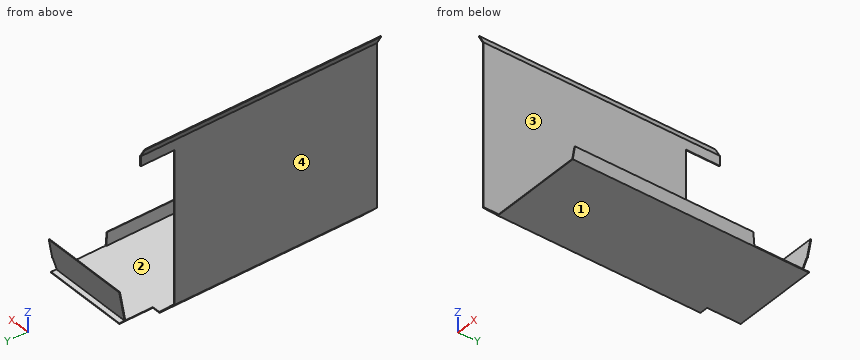
from build123d import *

# Parameters (mm, degrees)
F1_DEPTH  = 1076
F2_W      = 123
F2_H      = 775
F3_DEPTH  = 153
F5_DEPTH  = 402
F7_DEPTH  = 25
F9_DEPTH  = 50
F11_DEPTH = 260


with BuildPart() as f1:
    # F0 (on Front) → F1 (new body)
    with BuildSketch(Plane.XZ):
        Polygon((0, 819), (0, 85), (85, 0), (512, 0), (525, 50), (521.9029679783, 50.8052283256), (509.5256086136, 3.2), (86.3254833996, 3.2), (3.2, 86.3254833996), (3.2, 819.8498061986), (-21.2216219452, 862.5876446027), (-24, 861), align=None)
    extrude(amount=F1_DEPTH)

    # F2 (on face) → F3 (cut)
    with BuildSketch(Plane(origin=(0, 0, 0), x_dir=(-1, 0, 0), z_dir=(0, 1, 0))):
        with Locations((-61.5, 387.5)):
            Rectangle(F2_W, F2_H)
    extrude(amount=-F3_DEPTH, mode=Mode.SUBTRACT)

    # F4 (on face) → F5 (join)
    with BuildSketch(Plane(origin=(123, 0, 0), x_dir=(0, -1, 0), z_dir=(-1, 0, 0))):
        Polygon((0, 140), (25, 0), (28.1501682416, 0.5625300431), (3.1501682416, 140.5625300431), align=None)
    extrude(amount=-F5_DEPTH)

    # F6 (on face) → F7 (cut)
    with BuildSketch(Plane(origin=(476.483335157, 0, -123.8856671408), x_dir=(0, -1, 0), z_dir=(-0.9678225068, 0, 0.2516338518))):
        Polygon((15.927637799, 180.498897516), (24.4285714286, 131.31092349), (27.6760096229, 131.31092349), (19.1750759933, 180.498897516), align=None)
        Polygon((19.1750759933, 180.498897516), (27.6760096229, 131.31092349), (249, 131.31092349), (263.7563922078, 180.498897516), align=None)
        Polygon((0, 180.498897516), (0, 131.31092349), (24.4285714286, 131.31092349), (15.927637799, 180.498897516), align=None)
    extrude(amount=-F7_DEPTH, mode=Mode.SUBTRACT)

    # F8 (on face) → F9 (cut)
    with BuildSketch(Plane(origin=(0, 0, 0), x_dir=(-1, 0, 0), z_dir=(0, 1, 0))):
        Polygon((-525.584936142, 0), (-512, 0), (-513.4268980016, 5.488069237), align=None)
    extrude(amount=-F9_DEPTH, mode=Mode.SUBTRACT)

    # F10 (on face) → F11 (join)
    with BuildSketch(Plane(origin=(0, 0, 0), x_dir=(-1, 0, 0), z_dir=(0, 1, 0))):
        Polygon((-512.6226406353, 2.3947716744), (-509.5256086136, 3.2), (-512.6226406353, 3.2), align=None)
    extrude(amount=-F11_DEPTH)


solid = f1.part
Could you check a few things on this model? Use its own coordinates, in mm. Face numbers are marked on the shaded views. Round coordinates to 2 decimals unless told otherwise and drop trailing zeros. Order: outer loops, then holes, each group sorted by start corner. A loop starts at its lowest first (then second) coordinate and runs counter-clockwise, first axis right, second up. Notation, with made-up numbers: M 70.5,7.5 L 87.5,7.5 A24 cw 87.5,28.5 Z; hole C 14,-16.5 d2. An arc over 180 degrees is marked long. One line per item, written item: value.
(1) I'm going to push flat-ended pins straight in: P1, Ø4, axis at y = -839, z = 449, coming from the -X side; P2, Ø4, axis at x = 101, y = -584, coming from the +Z side; P3, Ø1, axis at x = 282, y = -196.5, coming from the -Z side; P4, Ø3.5, axis at x = 2.5, y = -114.5, coming from the -Z side. Where does each tip first touch, or does it pass through?
Ans:
P1: stops at x = 0
P2: stops at z = 3.2
P3: stops at z = 0
P4: stops at z = 775
(2) Imagine slicing it at B-B (y = -441.5). Write out the boundary of the cut face in (x, z), and give its area (3 significant figures).
Ans:
outline: M -24,861 L 0,819 L 0,85 L 85,0 L 512,0 L 525,50 L 521.9,50.81 L 509.53,3.2 L 86.33,3.2 L 3.2,86.33 L 3.2,819.85 L -21.22,862.59 Z
area: 4,410 mm^2
(3) Imagine slicing it at D-D (y = -205). Write out the boundary of the cut face in (x, z), and give its area (3 significant figures).
Ans:
outline: M -24,861 L 0,819 L 0,85 L 85,0 L 512,0 L 512.62,2.39 L 512.62,3.2 L 86.33,3.2 L 3.2,86.33 L 3.2,819.85 L -21.22,862.59 Z
area: 4,250 mm^2
(4) Imagine slicing it at A-A (x = 275). Write out the boundary of the cut face in (y, z), and give its area (3 significant figures).
Ans:
outline: M -1076,0 L 0,0 L 0,3.2 L -24.43,3.2 L 0,140 L -3.15,140.56 L -27.68,3.2 L -1076,3.2 Z
area: 3,890 mm^2
(5) Imagine slicing it at C-C (z = 107). Write out the boundary of the cut face in (x, y), and give its area (3 significant figures).
Ans:
outline: M 0,-1076 L 3.2,-1076 L 3.2,-153 L 0,-153 Z; M 123,-9.14 L 525,-9.14 L 525,-5.89 L 123,-5.89 Z
area: 4,260 mm^2
(6) If we mould it in two halves opening along X, with no side actions, what happens to the marked faces 1, 2, 3 and 4? For each: released by +X, released by -X, zero draft, split by the parting line, or undercut.
Ans:
face 1: zero draft
face 2: undercut
face 3: released by +X
face 4: released by -X
(7) I need wall thicknesses on line 1 along X through (y, z) = (-554.5, 572); line 2 along Y through (x, z) = (354, 114.5). Which ranges of each line are inside material? Lowest first, please. Write a range as from..to.
Ans:
line 1: x = 0..3.2
line 2: y = -7.8..-4.55
